Can you work these out from the model? Positions are in its coordinate system, mm. Face numbers are marked on the shaded views. Round coordinates to 2 decimals unless told otherwise and drop trailing zeros. Order: outer loops, then holes, each group sorted by start corner. A loop starts at its lowest first (then second) coordinate and runs counter-clockwise, first axis right, second up. Notation, with made-up numbers: M 72,-31 L 99,-31 A22 ccw 99,-2 Z; hole C 47.5,66 d4. An arc over 180 degrees is marked long. Answer as a JSON object with one key per item and string values. Group by question number.
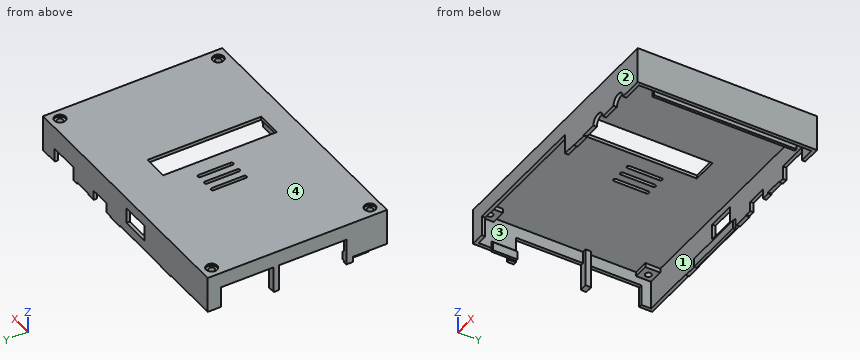
from build123d import *

# Parameters (mm, degrees)
SKETCH1_W               = 120.6
SKETCH1_H               = 80.6
BOSS_EXTRUDE1_DEPTH     = 1.6
SKETCH2_W               = 123.8
SKETCH2_H               = 83.8
BOSS_EXTRUDE2_DEPTH     = 1.6
SKETCH15_W              = 54.6
SKETCH15_H              = 1.6
BOSS_EXTRUDE10_DEPTH    = 15.4
SKETCH16_R              = 3.55
CUT_EXTRUDE5_DEPTH      = 15.5
BOSS_EXTRUDE11_DEPTH    = 15.4
SKETCH18_W              = 1.6
SKETCH18_H              = 3.2
SKETCH18_H_2            = 2.6
BOSS_EXTRUDE12_DEPTH    = 18
BOSS_EXTRUDE13_DEPTH    = 15.4
SKETCH20_W              = 15
SKETCH20_H              = 1.6
BOSS_EXTRUDE14_DEPTH    = 15.4
BOSS_EXTRUDE15_DEPTH    = 15.4
SKETCH22_W              = 62.6
SKETCH22_H              = 1.6
BOSS_EXTRUDE16_DEPTH    = 6
SKETCH23_W              = 1.6
SKETCH23_H              = 31.4
BOSS_EXTRUDE17_DEPTH    = 5.6
SKETCH24_W              = 1.6
SKETCH24_H              = 24.7
BOSS_EXTRUDE18_DEPTH    = 5.6
SKETCH25_W              = 11.5
SKETCH25_H              = 1.6
BOSS_EXTRUDE19_DEPTH    = 10.8
SKETCH26_W              = 14.3
SKETCH26_H              = 1.6
BOSS_EXTRUDE20_DEPTH    = 9
SKETCH27_W              = 8.4
SKETCH27_H              = 1.6
CUT_EXTRUDE6_DEPTH      = 0.6
SKETCH29_W              = 7
SKETCH29_H              = 7
BOSS_EXTRUDE21_DEPTH    = 2
CUT_EXTRUDE8_DEPTH      = 77.884458768
CUT_EXTRUDE8_DEPTH_BACK = 77.884458768
SKETCH28_R              = 1.4
SKETCH30_R              = 2.6
CUT_EXTRUDE9_DEPTH      = 1
SKETCH31_W              = 11.8
SKETCH31_H              = 53.2
CUT_EXTRUDE11_DEPTH     = 78.274704788
SKETCH32_W              = 13.6
SKETCH32_H              = 7.4
CUT_EXTRUDE12_DEPTH     = 10
SKETCH34_W              = 7.2
SKETCH34_H              = 1.6
BOSS_EXTRUDE22_DEPTH    = 0.4
SKETCH35_W              = 7.2
SKETCH35_H              = 1.6
BOSS_EXTRUDE23_DEPTH    = 0.4
SKETCH36_W              = 4
SKETCH36_H              = 66.6
BOSS_EXTRUDE25_DEPTH    = 1.2
SKETCH37_W              = 4
SKETCH37_H              = 11.4
BOSS_EXTRUDE31_DEPTH    = 1.2
SKETCH37_2_W            = 4
SKETCH37_2_H            = 11.4
BOSS_EXTRUDE36_DEPTH    = 1.2
SKETCH37_3_W            = 4
SKETCH37_3_H            = 11.4
BOSS_EXTRUDE37_DEPTH    = 1.2
SKETCH38_W              = 29.4
SKETCH38_H              = 4
BOSS_EXTRUDE40_DEPTH    = 1.2
CHAMFER1_SIZE           = 1.2
SKETCH39_W              = 18
SKETCH39_H              = 2.6
BOSS_EXTRUDE41_DEPTH    = 2


with BuildPart() as part:
    # Sketch1 → Boss-Extrude1 (new body)
    with BuildSketch(Plane.XY):
        Rectangle(SKETCH1_W, SKETCH1_H)
    extrude(amount=BOSS_EXTRUDE1_DEPTH)

    # Sketch2 → Boss-Extrude2 (add)
    with BuildSketch(Plane.XY):
        Rectangle(SKETCH2_W, SKETCH2_H)
    extrude(amount=BOSS_EXTRUDE2_DEPTH)

    # Sketch15 → Boss-Extrude10 (add)
    with BuildSketch(Plane(origin=(0, 0, 0), x_dir=(-1, 0, 0), z_dir=(0, 0, -1))):
        with Locations((-34.6, -41.1)):
            Rectangle(SKETCH15_W, SKETCH15_H)
    extrude(amount=BOSS_EXTRUDE10_DEPTH)

    # Sketch16 → Cut-Extrude5 (cut)
    with BuildSketch(Plane.XZ.offset(41.9)):
        with Locations((47.3, -15.4)):
            Circle(SKETCH16_R)
        with Locations((32.1, -15.4)):
            Circle(SKETCH16_R)
    extrude(amount=-CUT_EXTRUDE5_DEPTH, mode=Mode.SUBTRACT)

    # Sketch17 → Boss-Extrude11 (add)
    with BuildSketch(Plane(origin=(0, 0, 0), x_dir=(-1, 0, 0), z_dir=(0, 0, -1))):
        Polygon((55.3, -41.9), (61.9, -41.9), (61.9, -26.1), (60.3, -26.1), (60.3, -40.3), (55.3, -40.3), align=None)
    extrude(amount=BOSS_EXTRUDE11_DEPTH)

    # Sketch18 → Boss-Extrude12 (add)
    with BuildSketch(Plane(origin=(0, 0, 0), x_dir=(-1, 0, 0), z_dir=(0, 0, -1))):
        with Locations((61.1, -24.5)):
            Rectangle(SKETCH18_W, SKETCH18_H)
        with Locations((61.1, 9.8)):
            Rectangle(SKETCH18_W, SKETCH18_H_2)
    extrude(amount=BOSS_EXTRUDE12_DEPTH)

    # Sketch19 → Boss-Extrude13 (add)
    with BuildSketch(Plane(origin=(0, 0, 0), x_dir=(-1, 0, 0), z_dir=(0, 0, -1))):
        Polygon((60.3, 35.8), (61.9, 35.8), (61.9, 41.9), (-14.3, 41.9), (-14.3, 40.3), (60.3, 40.3), align=None)
    extrude(amount=BOSS_EXTRUDE13_DEPTH)

    # Sketch20 → Boss-Extrude14 (add)
    with BuildSketch(Plane(origin=(0, 0, 0), x_dir=(-1, 0, 0), z_dir=(0, 0, -1))):
        with Locations((-31.3, 41.1)):
            Rectangle(SKETCH20_W, SKETCH20_H)
    extrude(amount=BOSS_EXTRUDE14_DEPTH)

    # Sketch21 → Boss-Extrude15 (add)
    with BuildSketch(Plane(origin=(0, 0, 0), x_dir=(-1, 0, 0), z_dir=(0, 0, -1))):
        Polygon((-53.1, 40.3), (-53.1, 41.9), (-61.9, 41.9), (-61.9, -40.3), (-60.3, -40.3), (-60.3, 40.3), align=None)
    extrude(amount=BOSS_EXTRUDE15_DEPTH)

    # Sketch22 → Boss-Extrude16 (add)
    with BuildSketch(Plane(origin=(0, 0, 0), x_dir=(-1, 0, 0), z_dir=(0, 0, -1))):
        with Locations((24, -41.1)):
            Rectangle(SKETCH22_W, SKETCH22_H)
    extrude(amount=BOSS_EXTRUDE16_DEPTH)

    # Sketch23 → Boss-Extrude17 (add)
    with BuildSketch(Plane(origin=(0, 0, 0), x_dir=(-1, 0, 0), z_dir=(0, 0, -1))):
        with Locations((61.1, -7.2)):
            Rectangle(SKETCH23_W, SKETCH23_H)
    extrude(amount=BOSS_EXTRUDE17_DEPTH)

    # Sketch24 → Boss-Extrude18 (add)
    with BuildSketch(Plane(origin=(0, 0, 0), x_dir=(-1, 0, 0), z_dir=(0, 0, -1))):
        with Locations((61.1, 23.45)):
            Rectangle(SKETCH24_W, SKETCH24_H)
    extrude(amount=BOSS_EXTRUDE18_DEPTH)

    # Sketch25 → Boss-Extrude19 (add)
    with BuildSketch(Plane(origin=(0, 0, 0), x_dir=(-1, 0, 0), z_dir=(0, 0, -1))):
        with Locations((-19.65, 41.1)):
            Rectangle(SKETCH25_W, SKETCH25_H)
    extrude(amount=BOSS_EXTRUDE19_DEPTH)

    # Sketch26 → Boss-Extrude20 (add)
    with BuildSketch(Plane(origin=(0, 0, 0), x_dir=(-1, 0, 0), z_dir=(0, 0, -1))):
        with Locations((-45.95, 41.1)):
            Rectangle(SKETCH26_W, SKETCH26_H)
    extrude(amount=BOSS_EXTRUDE20_DEPTH)

    # Sketch27 → Cut-Extrude6 (cut)
    with BuildSketch(Plane(origin=(0, 0, -15.4), x_dir=(-1, 0, 0), z_dir=(0, 0, -1))):
        with Locations((-32, 41.1)):
            Rectangle(SKETCH27_W, SKETCH27_H)
    extrude(amount=-CUT_EXTRUDE6_DEPTH, mode=Mode.SUBTRACT)

    # Sketch29 → Boss-Extrude21 (add)
    with BuildSketch(Plane(origin=(0, 0, 0), x_dir=(-1, 0, 0), z_dir=(0, 0, -1))):
        with Locations((-56.8, -36.8)):
            Rectangle(SKETCH29_W, SKETCH29_H)
        with Locations((-56.8, 36.8)):
            Rectangle(SKETCH29_W, SKETCH29_H)
        with Locations((56.8, 36.8)):
            Rectangle(SKETCH29_W, SKETCH29_H)
        with Locations((56.8, -36.8)):
            Rectangle(SKETCH29_W, SKETCH29_H)
    extrude(amount=BOSS_EXTRUDE21_DEPTH)

    # Sketch28 → Cut-Extrude8 (cut, two sides: drawn at the far end of the back side and taken through both)
    with BuildSketch(Plane(origin=(0, 0, 0), x_dir=(-1, 0, 0), z_dir=(0, 0, -1)).offset(-CUT_EXTRUDE8_DEPTH_BACK)):
        with Locations((-57, 37)):
            Circle(SKETCH28_R)
        with Locations((57, 37)):
            Circle(SKETCH28_R)
        with Locations((57, -37)):
            Circle(SKETCH28_R)
        with Locations((-57, -37)):
            Circle(SKETCH28_R)
    extrude(amount=CUT_EXTRUDE8_DEPTH + CUT_EXTRUDE8_DEPTH_BACK, mode=Mode.SUBTRACT)

    # Sketch30 → Cut-Extrude9 (cut)
    with BuildSketch(Plane.XY.offset(1.6)):
        with Locations((-57, 37)):
            Circle(SKETCH30_R)
        with Locations((57, 37)):
            Circle(SKETCH30_R)
        with Locations((57, -37)):
            Circle(SKETCH30_R)
        with Locations((-57, -37)):
            Circle(SKETCH30_R)
    extrude(amount=-CUT_EXTRUDE9_DEPTH, mode=Mode.SUBTRACT)

    # Sketch31 → Cut-Extrude11 (cut, through all)
    with BuildSketch(Plane.XY.offset(1.6)):
        with Locations((10, -4.9)):
            Rectangle(SKETCH31_W, SKETCH31_H)
        with BuildLine():
            Line((-8.1, 9.7), (-8.1, -5.3))
            ThreePointArc((-8.1, -5.3), (-8.9, -6.1), (-9.7, -5.3))
            Line((-9.7, -5.3), (-9.7, 9.7))
            ThreePointArc((-9.7, 9.7), (-8.9, 10.5), (-8.1, 9.7))
        make_face()
        with BuildLine():
            Line((-13.1, 9.7), (-13.1, -5.3))
            ThreePointArc((-13.1, -5.3), (-13.9, -6.1), (-14.7, -5.3))
            Line((-14.7, -5.3), (-14.7, 9.7))
            ThreePointArc((-14.7, 9.7), (-13.9, 10.5), (-13.1, 9.7))
        make_face()
        with BuildLine():
            Line((-3.1, 9.7), (-3.1, -5.3))
            ThreePointArc((-3.1, -5.3), (-3.9, -6.1), (-4.7, -5.3))
            Line((-4.7, -5.3), (-4.7, 9.7))
            ThreePointArc((-4.7, 9.7), (-3.9, 10.5), (-3.1, 9.7))
        make_face()
    extrude(amount=-CUT_EXTRUDE11_DEPTH, mode=Mode.SUBTRACT)

    # Sketch32 → Cut-Extrude12 (cut)
    with BuildSketch(Plane(origin=(0, 41.9, 0), x_dir=(1, 0, 0), z_dir=(0, 1, 0))):
        with Locations((-7.6, 7.1)):
            Rectangle(SKETCH32_W, SKETCH32_H)
    extrude(amount=-CUT_EXTRUDE12_DEPTH, mode=Mode.SUBTRACT)

    # Sketch34 → Boss-Extrude22 (add)
    with BuildSketch(Plane(origin=(0, 0, -15.4), x_dir=(-1, 0, 0), z_dir=(0, 0, -1))):
        with Locations((-7.7, 41.1)):
            Rectangle(SKETCH34_W, SKETCH34_H)
        with Locations((30.5, 41.1)):
            Rectangle(SKETCH34_W, SKETCH34_H)
    extrude(amount=BOSS_EXTRUDE22_DEPTH)

    # Sketch35 → Boss-Extrude23 (add)
    with BuildSketch(Plane(origin=(0, 0, -15.4), x_dir=(-1, 0, 0), z_dir=(0, 0, -1))):
        with Locations((-17.7, -41.1)):
            Rectangle(SKETCH35_W, SKETCH35_H)
    extrude(amount=BOSS_EXTRUDE23_DEPTH)

    # Sketch36 → Boss-Extrude25 (add)
    with BuildSketch(Plane.ZY.offset(-60.3)):
        with Locations((-15.4, 0)):
            Rectangle(SKETCH36_W, SKETCH36_H)
    extrude(amount=BOSS_EXTRUDE25_DEPTH)

    # Sketch37 → Boss-Extrude31 (add)
    with BuildSketch(Plane(origin=(-60.3, 0, 0), x_dir=(0, 0, -1), z_dir=(1, 0, 0))):
        with Locations((15.317328584, -28.6)):
            Rectangle(SKETCH37_W, SKETCH37_H)
    extrude(amount=BOSS_EXTRUDE31_DEPTH)

    # Sketch37<2> → Boss-Extrude36 (add)
    with BuildSketch(Plane(origin=(-60.3, 0, 0), x_dir=(0, 0, -1), z_dir=(1, 0, 0))):
        with Locations((15.317328584, -28.6)):
            Rectangle(SKETCH37_2_W, SKETCH37_2_H)
    extrude(amount=BOSS_EXTRUDE36_DEPTH)

    # Sketch37<3> → Boss-Extrude37 (add)
    with BuildSketch(Plane(origin=(-60.3, 0, 0), x_dir=(0, 0, -1), z_dir=(1, 0, 0))):
        with Locations((15.317328584, -28.6)):
            Rectangle(SKETCH37_3_W, SKETCH37_3_H)
    extrude(amount=BOSS_EXTRUDE37_DEPTH)

    # Sketch38 → Boss-Extrude40 (add)
    with BuildSketch(Plane.XZ.offset(-40.3)):
        with Locations((-11.3, -15.4)):
            Rectangle(SKETCH38_W, SKETCH38_H)
    extrude(amount=BOSS_EXTRUDE40_DEPTH)

    # Chamfer1
    chamfer1_edges = [part.edges().sort_by_distance(p)[0] for p in [
        (60.3, 0, -13.4),
        (-60.3, -28.6, -13.317328584),
        (-11.3, 40.3, -13.4),
    ]]
    chamfer(chamfer1_edges, length=CHAMFER1_SIZE - 0.0001)  # a hair under: the kernel refuses the full size

    # Sketch39 → Boss-Extrude41 (add)
    with BuildSketch(Plane(origin=(-60.3, 0, 0), x_dir=(0, 0, -1), z_dir=(1, 0, 0))):
        with Locations((9, 9.8)):
            Rectangle(SKETCH39_W, SKETCH39_H)
    extrude(amount=BOSS_EXTRUDE41_DEPTH)


solid = part.part
Item 1: I'm going to push flat-ended pins straight in: pin 1 Ø5 at (x, y) = (27, 27.5) entering from -Z; pin 2 Ø0.5 at (x, y) = (-29.5, 40.5) entering from -Z; pin 3 Ø0.5 at (x, y) = (-8, 41) entering from -Z. Where does each tip first touch, or does it pass through?
Item 2: I need wall thicknesses on line 1 (Y direction, x = 57, z = -1.4); line 2 (Y direction, x = 26, z = -4); line 3 (Y direction, x = 57, z = 0.5). Which ranges of each line are inside material? Lowest first, please.
Item 3: Suppose I cut it at B-B, the plane y = -37. Write out the boundary of the cut face in (x, z), and give its area (3 significant figures).
Item 4: Suppose I cut it at C-C, the plane x = -35.5. Write out the boundary of the cut face in (y, z), and give its area (3 significant figures).
Item 5: If we mould it in two halves opening along Z, with no side actions, what happens to the marked faces 1, 2, 3 and 4? For each: +Z half, -Z half, draft (parallel to the pull), parting line (faces both ways), or undercut.
Item 6: Suppose I cut it at A-A, the plane z = -7.5. Write out the boundary of the cut face in (x, y).
Item 7: Suppose I cut it at D-D, the plane y = -1.5. State how many separate pieces and enclosed holes the cut face has, and give its area (3 significant figures).
Computed:
{
 "1": {"pin 1": "stops at z = 0", "pin 2": "stops at z = -15.8", "pin 3": "stops at z = -15.4"},
 "2": {"line 1": "y = -41.9 to -38.4, -35.6 to -33.3, 33.3 to 35.6, 38.4 to 41.9", "line 2": "y = -41.9 to -40.3, 40.3 to 41.9", "line 3": "y = -41.9 to -38.4, -35.6 to 35.6, 38.4 to 41.9"},
 "3": {"outline": "M -61.9,-15.4 L -60.3,-15.4 L -60.3,-2 L -58.4,-2 L -58.4,0.6 L -59.6,0.6 L -59.6,1.6 L -61.9,1.6 Z; M -55.6,-2 L -53.3,-2 L -53.3,0 L 53.3,0 L 53.3,-2 L 55.6,-2 L 55.6,0.6 L 54.4,0.6 L 54.4,1.6 L -54.4,1.6 L -54.4,0.6 L -55.6,0.6 Z; M 58.4,-2 L 60.3,-2 L 60.3,-15.4 L 61.9,-15.4 L 61.9,1.6 L 59.6,1.6 L 59.6,0.6 L 58.4,0.6 Z", "area": "250 mm^2"},
 "4": {"outline": "M -41.9,-6 L -40.3,-6 L -40.3,0 L 40.3,0 L 40.3,-15.4 L 41.9,-15.4 L 41.9,1.6 L -41.9,1.6 Z", "area": "168 mm^2"},
 "5": {"face 1": "undercut", "face 2": "draft", "face 3": "undercut", "face 4": "+Z half"},
 "6": {"outline": "M -61.9,-41.9 L -55.3,-41.9 L -55.3,-40.3 L -60.3,-40.3 L -60.3,-22.9 L -61.9,-22.9 Z; M -61.9,8.5 L -58.3,8.5 L -58.3,11.1 L -61.9,11.1 Z; M -61.9,35.8 L -60.3,35.8 L -60.3,40.3 L -14.4,40.3 L -14.4,41.9 L -61.9,41.9 Z; M -0.8,40.3 L 60.3,40.3 L 60.3,-40.3 L 7.3,-40.3 L 7.3,-41.9 L 61.9,-41.9 L 61.9,41.9 L -0.8,41.9 Z"},
 "7": {"separate pieces": "5", "enclosed holes": "0", "area": "211 mm^2"}
}
